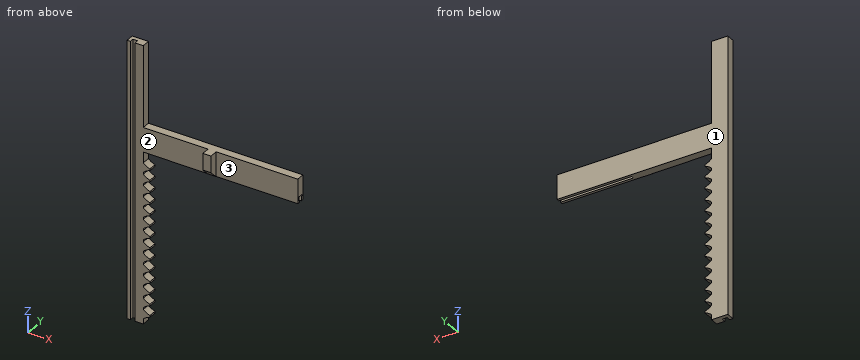
Autodesk Inventor part; units mm, degrees
ref_plane "YZ Plane" through (0, 0, 0) normal (1, 0, 0) x (0, 1, 0)
ref_plane "XZ Plane" through (0, 0, 0) normal (0, 1, 0) x (-1, 0, 0)
ref_plane "XY Plane" through (0, 0, 0) normal (0, 0, 1) x (1, 0, 0)
sketch "Sketch1" plane through (0, 0, 0) normal (0, 1, 0) x (-1, 0, 0)
  line L0 (0, 0) -> (10, 0)
  line L1 (10, 0) -> (10, -170)
  line L2 (10, -170) -> (0, -170)
  line L3 (0, -170) -> (0, 0)
  dimension "d0" = 170
  dimension "d1" = 10
extrude "Extrusion1" add sketch "Sketch1" along normal blind 5
sketch "Sketch2" plane through (-10, 0, 0) normal (0, 0, 1) x (1, 0, 0)
  line L0 (2, 0) -> (2, 2.5)
  line L1 (2, 2.5) -> (5, 2.5)
  line L2 (0, 0) -> (0, 5)
  line L3 (5, 2.5) -> (5, 0)
  line L4 (0, 0) -> (10, 0)
  dimension "d6" = 2
  dimension "d9" = 3
  dimension "d75" = 2.5
sketch "Sketch4" plane through (0, 5, 0) normal (0, 1, 0) x (1, 0, 0)
  line L0 (95.426, 50) -> (95.426, 65)
  line L1 (95.426, 65) -> (0, 65)
  line L2 (95.426, 50) -> (0, 50)
  line L3 (-10, 0) -> (0, 0)
  line L4 (0, 0) -> (0, 170)
  line L5 (0, 50) -> (0, 65)
  dimension "d107" = 95.426
  dimension "d108" = 15
  dimension "d109" = 50
extrude "Extrusion4" add sketch "Sketch4" against normal blind 5
sketch "Sketch6" plane through (0, 5, 0) normal (0, 1, 0) x (1, 0, 0)
  line L0 (0, 0) -> (0, 170)
  line L1 (95.426, 50) -> (95.426, 65)
  arc A0 (4.0959, 156.5581) -> (0, 154.1943) centre (6.5788, 147.5251) ccw
  arc A1 (4.0959, 157.6362) -> (4.0959, 156.5581) centre (9.5694, 157.0972) ccw
  arc A2 (0, 160) -> (4.0959, 157.6362) centre (6.5788, 166.6692) ccw
  line L2 (0, 154.1943) -> (0, 160)
  arc A3 (4.0959, 163.4421) -> (0, 161.0783) centre (6.5788, 154.4091) ccw
  arc A4 (4.0959, 164.5202) -> (4.0959, 163.4421) centre (9.5694, 163.9812) ccw
  arc A5 (0, 166.884) -> (4.0959, 164.5202) centre (6.5788, 173.5532) ccw
  arc A6 (4.0959, 149.6741) -> (0, 147.3103) centre (6.5788, 140.6411) ccw
  arc A7 (4.0959, 150.7522) -> (4.0959, 149.6741) centre (9.5694, 150.2132) ccw
  arc A8 (0, 153.116) -> (4.0959, 150.7522) centre (6.5788, 159.7852) ccw
  arc A9 (4.0959, 142.7901) -> (0, 140.4263) centre (6.5788, 133.7571) ccw
  arc A10 (4.0959, 143.8682) -> (4.0959, 142.7901) centre (9.5694, 143.3292) ccw
  arc A11 (0, 146.232) -> (4.0959, 143.8682) centre (6.5788, 152.9012) ccw
  arc A12 (4.0959, 135.9061) -> (0, 133.5423) centre (6.5788, 126.8731) ccw
  arc A13 (4.0959, 136.9842) -> (4.0959, 135.9061) centre (9.5694, 136.4452) ccw
  arc A14 (0, 139.348) -> (4.0959, 136.9842) centre (6.5788, 146.0172) ccw
  arc A15 (4.0959, 129.0221) -> (0, 126.6583) centre (6.5788, 119.9891) ccw
  arc A16 (4.0959, 130.1002) -> (4.0959, 129.0221) centre (9.5694, 129.5612) ccw
  arc A17 (0, 132.464) -> (4.0959, 130.1002) centre (6.5788, 139.1332) ccw
  arc A18 (4.0959, 122.1381) -> (0, 119.7743) centre (6.5788, 113.1051) ccw
  arc A19 (4.0959, 123.2162) -> (4.0959, 122.1381) centre (9.5694, 122.6772) ccw
  arc A20 (0, 125.58) -> (4.0959, 123.2162) centre (6.5788, 132.2492) ccw
  arc A21 (4.0959, 115.2541) -> (0, 112.8903) centre (6.5788, 106.2211) ccw
  arc A22 (4.0959, 116.3322) -> (4.0959, 115.2541) centre (9.5694, 115.7932) ccw
  arc A23 (0, 118.696) -> (4.0959, 116.3322) centre (6.5788, 125.3652) ccw
  arc A24 (4.0959, 108.3701) -> (0, 106.0063) centre (6.5788, 99.3371) ccw
  arc A25 (4.0959, 109.4482) -> (4.0959, 108.3701) centre (9.5694, 108.9092) ccw
  arc A26 (0, 111.812) -> (4.0959, 109.4482) centre (6.5788, 118.4812) ccw
  arc A27 (4.0959, 101.4861) -> (0, 99.1223) centre (6.5788, 92.4531) ccw
  arc A28 (4.0959, 102.5642) -> (4.0959, 101.4861) centre (9.5694, 102.0252) ccw
  arc A29 (0, 104.928) -> (4.0959, 102.5642) centre (6.5788, 111.5972) ccw
  arc A30 (4.0959, 94.6021) -> (0, 92.2383) centre (6.5788, 85.5691) ccw
  arc A31 (4.0959, 95.6802) -> (4.0959, 94.6021) centre (9.5694, 95.1412) ccw
  arc A32 (0, 98.044) -> (4.0959, 95.6802) centre (6.5788, 104.7132) ccw
  arc A33 (4.0959, 87.7181) -> (0, 85.3543) centre (6.5788, 78.6851) ccw
  arc A34 (4.0959, 88.7962) -> (4.0959, 87.7181) centre (9.5694, 88.2572) ccw
  arc A35 (0, 91.16) -> (4.0959, 88.7962) centre (6.5788, 97.8292) ccw
  arc A36 (4.0959, 80.8341) -> (0, 78.4703) centre (6.5788, 71.8011) ccw
  arc A37 (4.0959, 81.9122) -> (4.0959, 80.8341) centre (9.5694, 81.3732) ccw
  arc A38 (0, 84.276) -> (4.0959, 81.9122) centre (6.5788, 90.9452) ccw
  arc A39 (4.0959, 73.9501) -> (0, 71.5863) centre (6.5788, 64.9171) ccw
  arc A40 (4.0959, 75.0282) -> (4.0959, 73.9501) centre (9.5694, 74.4892) ccw
  arc A41 (0, 77.392) -> (4.0959, 75.0282) centre (6.5788, 84.0612) ccw
  point P0 (0, 65)
  point P1 (0, 154.1943)
  point P2 (0, 166.884)
  point P3 (0, 161.0783)
  point P4 (0, 77.392)
  point P5 (0, 71.5863)
  point P6 (0, 84.276)
  point P7 (0, 78.4703)
  point P8 (0, 91.16)
  point P9 (0, 85.3543)
  point P10 (0, 98.044)
  point P11 (0, 92.2383)
  point P12 (0, 104.928)
  point P13 (0, 99.1223)
  point P14 (0, 111.812)
  point P15 (0, 106.0063)
  point P16 (0, 118.696)
  point P17 (0, 112.8903)
  point P18 (0, 125.58)
  point P19 (0, 119.7743)
  point P20 (0, 132.464)
  point P21 (0, 126.6583)
  point P22 (0, 139.348)
  point P23 (0, 133.5423)
  point P24 (0, 146.232)
  point P25 (0, 140.4263)
  point P26 (0, 153.116)
  point P27 (0, 147.3103)
  dimension "d80" = 6.884
  dimension "d88" = 6.884
  dimension "d200" = 5.5
  dimension "d201" = 9.368
  dimension "d202" = 95.426
  dimension "d203" = 95.426
  dimension "d204" = 85.8566
  dimension "d205" = 88.8472
  dimension "d206" = 88.8472
  dimension "d207" = 91.3301
  dimension "d208" = 91.3301
  dimension "d209" = 95.426
  dimension "d210" = 95.426
  dimension "d211" = 95.426
  dimension "d212" = 95.426
  dimension "d213" = 95.426
  dimension "d214" = 95.426
  dimension "d215" = 95.426
  dimension "d216" = 95.426
  dimension "d217" = 95.426
  dimension "d218" = 95.426
  dimension "d219" = 95.426
  dimension "d220" = 95.426
  dimension "d221" = 95.426
  dimension "d222" = 95.426
  dimension "d223" = 95.426
  dimension "d224" = 95.426
  dimension "d225" = 95.426
  dimension "d226" = 95.426
  dimension "d227" = 95.426
  dimension "d228" = 95.426
  dimension "d229" = 95.426
  dimension "d230" = 95.426
  dimension "d231" = 95.426
  dimension "d232" = 95.426
  dimension "d233" = 95.426
  dimension "d234" = 95.426
  dimension "d235" = 95.426
  dimension "d236" = 95.426
  dimension "d237" = 131.0291
  dimension "d238" = 139.594
  dimension "d239" = 135.4148
  dimension "d240" = 134.6518
  dimension "d241" = 130.6206
  dimension "d242" = 129.8867
  dimension "d243" = 126.0203
  dimension "d244" = 125.3186
  dimension "d245" = 121.6357
  dimension "d246" = 120.97
  dimension "d247" = 117.4912
  dimension "d248" = 116.8654
  dimension "d249" = 113.6128
  dimension "d250" = 113.0312
  dimension "d251" = 110.0288
  dimension "d252" = 109.496
  dimension "d253" = 106.7689
  dimension "d254" = 106.2896
  dimension "d255" = 103.8636
  dimension "d256" = 103.4426
  dimension "d257" = 101.3432
  dimension "d258" = 100.9853
  dimension "d259" = 99.2373
  dimension "d260" = 98.9468
  dimension "d261" = 97.5726
extrude "Extrusion6" add sketch "Sketch6" against normal blind 5
extrude "Extrusion10" cut sketch "Sketch2" against normal blind 300
sketch "Sketch9" plane through (0, 0, 0) normal (0, -1, 0) x (1, 0, 0)
  line L0 (95.426, -65) -> (0, -65)
  line L1 (40, -50) -> (45, -50)
  line L2 (45, -50) -> (45, -65)
  line L3 (45, -65) -> (40, -65)
  line L4 (40, -65) -> (40, -50)
  line L5 (95.426, -50) -> (0, -50)
  line L6 (-10, -170) -> (-10, 0)
  point P0 (0, 0)
  dimension "d93" = 5
  dimension "d94" = 55
extrude "Extrusion11" add sketch "Sketch9" along normal blind 4.95
chamfer "Chamfer1" distance 4.75 angle 45 1 edges at (42.5, -4.95, -65)
sketch "Sketch11" plane through (95.426, 5, -50) normal (1, 0, 0) x (0, 0, -1)
  line L0 (15, 0) -> (15, -5)
  line L1 (11.5, -1) -> (11.5, -4)
  line L2 (11.5, -4) -> (15, -3.3829)
  line L3 (11.5, -1) -> (15, -1.6171)
  point P0 (11.5, -2.5)
  point P1 (15, -2.5)
  dimension "d100" = 3.5
  dimension "d101" = 80
  dimension "d104" = 3
extrude "Extrusion12" cut sketch "Sketch11" against normal blind 45
properties part number "Rack"
The model under review builds one solid part; all positions refer to its coordinate system, in mm. Face numbers are marked on the shaded views. A direction names the side the tool comes from. Give positions to 0.01 mm unless a question says otherwise; leave off trailing zeros. Write each loop counter-clockwise with the first axis right and the second up, starting at its lowest first coordinate (ties: lowest second). Pieces come first, ordered by that corner, then holes. Notation, with made-up numbers: (30, 76.5) -> (51, 76.5) arc R6 cw to (51, 84.5) -> close; hole circle Ø8 at (-18, -14). An arc over 180 degrees is marked (long way). Put each result on its own line as item: value.
(1) We need section A-A, the plane x = 55. Give the boundary of the cut face in (y, z), and give its area (3 significant figures).
Results are:
outline: (0, -65) -> (1.62, -65) -> (1, -61.5) -> (4, -61.5) -> (3.38, -65) -> (5, -65) -> (5, -50) -> (0, -50) -> close
area: 66.7 mm²
(2) For pin 1 Ø4 at (x, y) = (11.5, 0.5) entering from +Z; pin 2 Ø7.5 at (x, z) = (78.5, -59) entering from -Y; pin 3 Ø0.9 at (x, y) = (82, 2.5) entering from -Z, all flat-tipped, find the tip position at first contact; note any pin that passes through.
Results are:
pin 1: z = -50
pin 2: y = 0
pin 3: z = -61.5
(3) We need section D-D, the plane x = -3. Give the boundary of the cut face in (y, z).
Results are:
outline: (0, -170) -> (5, -170) -> (5, 0) -> (0, 0) -> close
(4) Tool access review of the marked faces 1, 2 and 3: name each direction out of +Z, -Z, +X, -X, +Y, -Y from which nothing blocks a thin tool from reaching the whole face with its end or side.
Results are:
face 1: +Z, -Z, +X, -X, +Y
face 2: +Z, -Z, -X, -Y
face 3: +Z, -Z, +X, -Y
(5) We need section C-C, the plane y = -2.25. Give the boundary of the cut face in (x, z), and give its area (4 significant figures).
Results are:
outline: (40, -62.95) -> (45, -62.95) -> (45, -50) -> (40, -50) -> close
area: 64.75 mm²
(6) To check wall thickness, follow probe 1 along X at (y, z) = (1, -29); probe 2 along Z at (x, y) = (75.5, 2.5); probe 3 along Z at (x, y) = (19, 1.25). State the ranges of each line that lie inside material, in increasing order. Write a range as from..to.
Results are:
probe 1: -10..-8, -5..0
probe 2: -61.5..-50
probe 3: -65..-50
(7) We need section B-B, the plane z = -14.5. Give the boundary of the cut face in (x, y), and give its area (3 significant figures).
Results are:
outline: (-10, 0) -> (-8, 0) -> (-8, 2.5) -> (-5, 2.5) -> (-5, 0) -> (0, 0) -> (0, 5) -> (-10, 5) -> close
area: 42.5 mm²
